```python
from build123d import *

# Parameters (mm, degrees)
F1_DEPTH     = 3.556
F2_R         = 12.7
F5_R         = 13.0437301263
F6_DEPTH     = 3.81
F7_R         = 12.7
F8_R         = 17.78
F10_DEPTH    = 8.382
F11_T1_DEPTH = 46.8316092758
F12_T1_DEPTH = 33.4229165443


# Not quite as in the source:
# - a fillet or chamfer that OpenCascade refuses, or shapes differently, is made with other operations: its cross-section is extruded or revolved along the edge and cut away or added
# - two fillets or chamfers of one size are made in one step


with BuildPart() as f1:
    # F0 (on Front) → F1 (new body)
    with BuildSketch(Plane.XZ):
        Polygon((-47.1675397517, 46.3941131987), (-32.3176106954, -28.3448967427), (26.3168609286, -28.3448967427), (41.4012483693, 46.3471460432), (32.0179715002, 54.9054236268), (-37.7416395402, 54.9054236268), align=None)
    extrude(amount=F1_DEPTH)

    # F2
    f2_edges = [f1.edges().sort_by_distance(p)[0] for p in [
        (-47.16754, -1.778, 46.394113),
        (41.401248, -1.778, 46.347146),
        (32.017972, -1.778, 54.905424),
        (-37.74164, -1.778, 54.905424),
    ]]
    fillet(f2_edges, radius=F2_R)

    # F5
    f5_edges = [f1.edges().sort_by_distance(p)[0] for p in [
        (26.316861, -1.778, -28.344897),
    ]]
    fillet(f5_edges, radius=F5_R)

    # F0 (on Front) → F6 (join)
    with BuildSketch(Plane.XZ):
        Polygon((26.3168609286, -28.3448967427), (-32.3176106954, -28.3448967427), (-17.7800003439, -40.6717509031), (12.8904990852, -40.6717509031), align=None)
        Polygon((-47.1675397517, 46.3941131987), (-32.3176106954, -28.3448967427), (26.3168609286, -28.3448967427), (41.4012483693, 46.3471460432), (32.0179715002, 54.9054236268), (-37.7416395402, 54.9054236268), align=None)
    extrude(amount=F6_DEPTH)

    # F7
    f7_edges = [f1.edges().sort_by_distance(p)[0] for p in [
        (32.017972, -1.905, 54.905424),
        (41.401248, -1.905, 46.347146),
        (-37.74164, -1.905, 54.905424),
        (-47.16754, -1.905, 46.394113),
    ]]
    fillet(f7_edges, radius=F7_R)

    # F8
    f8_edges = [f1.edges().sort_by_distance(p)[0] for p in [
        (-17.78, -1.905, -40.671751),
        (12.890499, -1.905, -40.671751),
        (26.316861, -1.905, -28.344897),
        (-32.317611, -1.905, -28.344897),
    ]]
    fillet(f8_edges, radius=F8_R)

    # F9 (on Right) → F10 (join)
    with BuildSketch(Plane.YZ):
        Polygon((-55.1818351742, -187.108784914), (-51.6164600849, -187.108784914), (-45.784432441, -183.5964620113), (2.1481101867, -34.6464961767), (-4.9838987179, -41.8398082256), align=None)
    extrude(amount=-F10_DEPTH)

    # F11: fillet of radius 9.6308354503 on 1 edges, made by hand

    # F11_s2 → F11_t1 (cut)
    with BuildSketch(Plane.YZ.offset(-27.6068046379)):
        with BuildLine():
            ThreePointArc((0, -36.813070433), (0.2476438249, -39.4040498919), (-0.2075604578, -41.9667225361))
            Line((-0.2075604578, -41.9667225361), (2.1481101867, -34.6464961767))
            Line((2.1481101867, -34.6464961767), (0, -36.813070433))
        make_face()
    extrude(amount=F11_T1_DEPTH, mode=Mode.SUBTRACT)

    # F12: fillet of radius 29.6825671573 on 1 edges, made by hand

    # F12_s2 → F12_t1 (cut)
    with BuildSketch(Plane.YZ.offset(-20.9024582721)):
        with BuildLine():
            ThreePointArc((-3.81, -40.6558192676), (-5.3785338271, -43.5368424871), (-6.6195826892, -46.5733521413))
            Line((-6.6195826892, -46.5733521413), (-4.9838987179, -41.8398082256))
            Line((-4.9838987179, -41.8398082256), (-3.81, -40.6558192676))
        make_face()
    extrude(amount=F12_T1_DEPTH, mode=Mode.SUBTRACT)


solid = f1.part
```
Input: part model. Units: mm. Frame: model coordinates. A direction names the side the tool comes from. Give positions to 0.01 mm unless a question says otherwise; leave off trailing zeros. Write each loop counter-clockwise with the first axis right and the second up, starting at its lowest first coordinate (ties: lowest second). Pieces come first, ordered by that corner, then holes. Notation, with made-up numbers: (-8, 35.5) - (5, 35.5) arc R28 ccw to (5, 58.5) - close; hole circle Ø10 at (-3.75, 33). An arc over 180 degrees is marked (long way). Write item = value, one per line. Start each with the question number.
1. First-contact query: pin 1 Ø4 at (x, y) = (4.5, -1) entering from -Z; pin 2 Ø10 at (x, z) = (-19, -35) entering from -Y; pin 3 Ø16.5 at (y, z) = (-25, -112) entering from -X. Flat tips, straight axial feed; report the tip coordinate or a pass-through.
2. Ray query, L1, parallel to Y at x = 9.5, z = -32.5; L2, parallel to Z at x = 1, y = -1.5; L3, parallel to X at y = -30, z = -126. Return the intervals inside material, ascending.
3. Section query B-B, the plane z = -140. Output: boundary loops of the cut face in (x, y).
4. Section query C-C, the plane y = -22.5. Output: boundary loops of the cut face in (x, z), then the cut area to 3 significant figures.
5. Access query for faces 1 (the flat face through (-4.132, -23.315, -113.773)), 2 (the flat face through (-3, -3.81, 8)). Directions: +Z, -Z, +X, -X, +Y, -Y. A direction counts if a zero-diameter tool reaches every point of the face in a straight line with its end or side. Return the directions, or none.
6. Section query A-A, the plane x = -5.5. Output: boundary loops of the cut face in (y, z), then the cut area to 3 significant figures.
Check sheet entries:
q1.pin_1 = -40.67
q1.pin_2 = -3.81
q1.pin_3 = -8.38
q2.L1 = -3.81 to 0
q2.L2 = -40.67 to 54.91
q2.L3 = -8.38 to 0
q3.outline = (-8.38, -38.9) - (0, -38.9) - (0, -31.75) - (-8.38, -31.75) - close
q4.outline = (-8.38, -111.24) - (0, -111.24) - (0, -92.53) - (-8.38, -92.53) - close
q4.area = 157 mm2
q5.face_1 = -Z, +X, -X, +Y
q5.face_2 = +Z, +X, -X, -Y
q6.outline = (-55.18, -187.11) - (-51.62, -187.11) - (-45.78, -183.6) - (-0.21, -41.97) arc R9.63 ccw to (0, -36.81) - (0, 54.91) - (-3.81, 54.91) - (-3.81, -40.66) arc R29.68 ccw to (-6.62, -46.57) - close
q6.area = 1,310 mm2
